Model file for the job. Use its own axes, mm. Coordinates: 2 decimals unless noted, no trailing zeros. Write each loop counter-clockwise with the first axis right and the second up, starting at its lowest first coordinate (ties: lowest second). Pieces come first, ordered by that corner, then holes.
Q1. Band-saw the part on B-B, the plane z = 795. Write the cut outline in (x, y).
Q2. Pin check, flat tips, straight feed: P1, Ø6, axis at y = 22.5, z = 819.5, coming from the +X side; P2, Ø5, axis at x = 51, y = 9, coming from the +Z side; P3, Ø24, axis at x = 44, z = 1835, coming from the -Y side. Stop position of each tip, or through.
Q3. Band-saw the part on A-A, the plane x = 24.5. Write the cut outline in (y, z), plus the area to 3 significant figures.
Q4. Drill centre lines: probe 1 along Y at (x, z) = (73, 1458); probe 2 along X at (y, z) = (11.5, 1488); probe 3 along Z at (x, y) = (26.5, 3). Where is each one in solid material? Low to high.
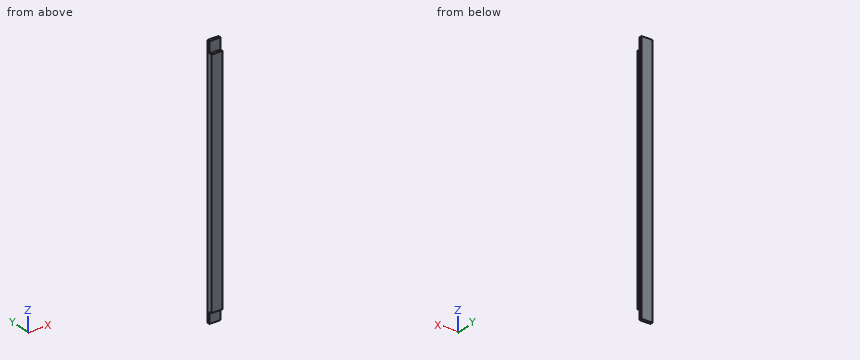
from build123d import *

# Parameters (mm, degrees)
F1_DEPTH = 80
F3_DEPTH = 12


with BuildPart() as f1:
    # F0 (on Right) → F1 (new body)
    with BuildSketch(Plane.YZ):
        Polygon((20, 86.632449), (20, 6.632449), (40, 6.632449), (40, 1861.632449), (20, 1861.632449), (20, 1781.632449), (0, 1781.632449), (0, 86.632449), align=None)
    extrude(amount=F1_DEPTH)

    # F2 (on face) → F3 (cut)
    with BuildSketch(Plane.YZ.offset(80)):
        Polygon((20, 1781.632449), (10, 1781.632449), (10, 86.632449), (20, 86.632449), (30, 86.632449), (30, 1781.632449), align=None)
    extrude(amount=-F3_DEPTH, mode=Mode.SUBTRACT)


solid = f1.part
Answer sheet:
1. outline: (0, 0) - (80, 0) - (80, 10) - (68, 10) - (68, 30) - (80, 30) - (80, 40) - (0, 40) - close
2. P1: stops at x = 68
2. P2: stops at z = 1781.63
2. P3: stops at y = 20
3. outline: (0, 86.63) - (20, 86.63) - (20, 6.63) - (40, 6.63) - (40, 1861.63) - (20, 1861.63) - (20, 1781.63) - (0, 1781.63) - close
3. area: 71,000 mm2
4. probe 1: y = 0 to 10, 30 to 40
4. probe 2: x = 0 to 68
4. probe 3: z = 86.63 to 1781.63
